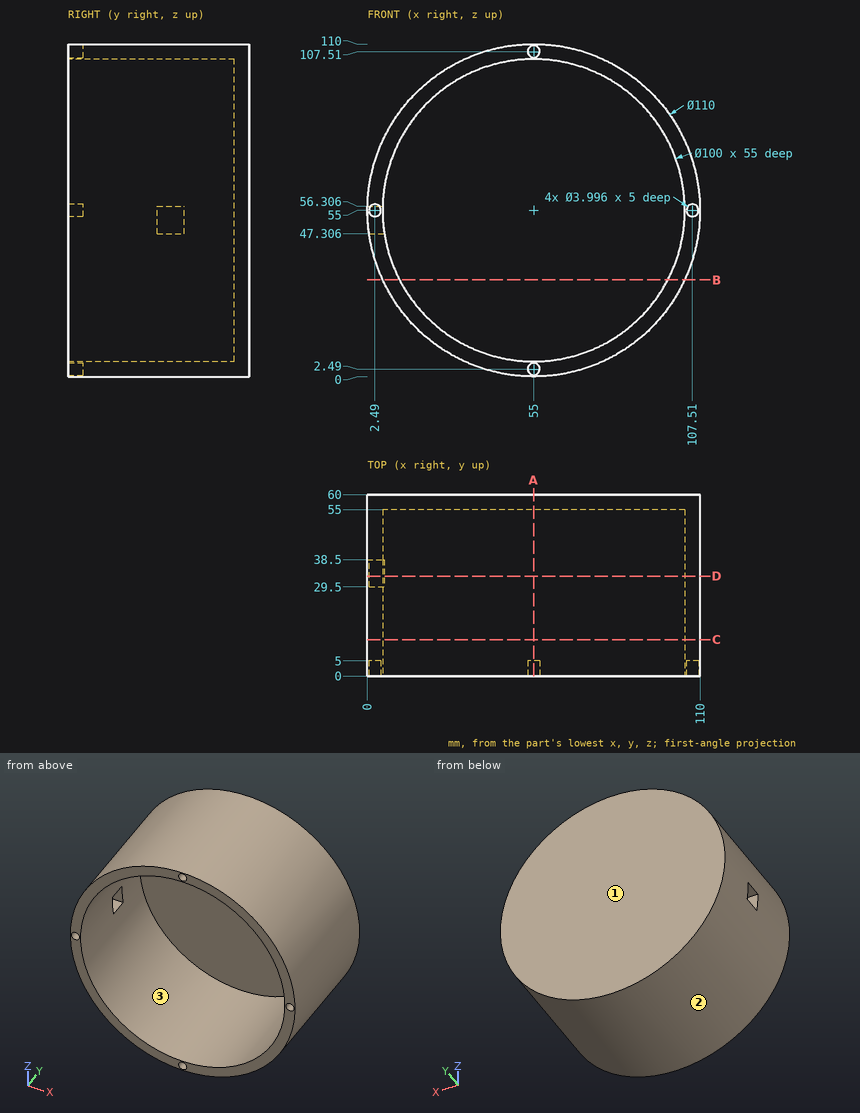
Answer from the drawing. Dimensions are ordinates in mm from the lowest x, y and z of the part. Coordinates: 2 decimals unless noted, no trailing zeros. Loops run counter-clockwise (first coordinate to the right, second up) from the corner with the lowest first, then second, coordinate; pieces in that order, holes last.
1) Section A-A (x = 55) is taken. Give the vertices of the cut face in (y, z), plus the area to 3 significant figures.
Results:
outline: (0, 0) - (60, 0) - (60, 110) - (0, 110) - (0, 109.51) - (5, 109.51) - (5, 105.51) - (0, 105.51) - (0, 105) - (55, 105) - (55, 5) - (0, 5) - (0, 4.49) - (5, 4.49) - (5, 0.49) - (0, 0.49) - close
area: 1,060 mm2
2) For a pull along X with two mould halves and no side action, classify the marked faces 1, 2 and 3 as +X half, -X half, draft (parallel to the pull), parting line (faces both ways), or undercut.
Results:
face 1: draft
face 2: parting line
face 3: undercut
3) Section D-D (y = 33) is taken. Give the vertices of the cut face in (x, z) (1 decimal), plus the area to 3 significant figures.
Results:
outline: (0, 56.3) - (5, 56.3) arc R50 cw (long way) to (5.6, 47.3) - (0.5, 47.3) arc R55 ccw (long way) to start
area: 1,600 mm2
4) Section C-C (y = 12) is taken. Give the vertices of the cut face in (x, z).
Results:
outline: circle Ø110 at (55, 55); hole circle Ø100 at (55, 55)
5) Section B-B (z = 32) is taken. Give the vertices of the cut face in (x, y), plus the area to 3 significant figures.
Results:
outline: (5.04, 0) - (10.6, 0) - (10.6, 55) - (99.4, 55) - (99.4, 0) - (104.96, 0) - (104.96, 60) - (5.04, 60) - close
area: 1,110 mm2
6) Consider probe 1 along Y at (x, z) = (46.5, 42.5); probe 2 along Z at (x, y) = (49.5, 4.5) (1 decimal); probe 3 along Z at (x, y) = (80.5, 7). Determine where each line is inside the solid, lowest interval first.
Results:
probe 1: y = 55 to 60
probe 2: z = 0.3 to 5.3, 104.7 to 109.7
probe 3: z = 6.27 to 11.99, 98.01 to 103.73
7) Flat-ended cylindrical pins translate along their axes: pin 1 (4 mm diameter, centred on x = 28, y = 42.5, fed in from -Z); pin 2 (12 mm diameter, centred on x = 55.5, z = 61, fed in from -Y); pin 3 (5 mm diameter, centred on x = 89, y = 22, fed in from +Z) (1 decimal); pin 4 (6 mm diameter, centred on x = 2.5, z = 53.5, fed in from -Y). Find the tip coordinate at first contact, or state that the pin passes through.
Results:
pin 1: stops at z = 6.01
pin 2: stops at y = 55
pin 3: stops at z = 100.1
pin 4: stops at y = 0
